Read the model definition and answer for the solid it produces. Units are mm, in the model's axes. A direction names the side the tool comes from. Give positions to 0.01 mm unless a question says otherwise; leave off trailing zeros. Loops run counter-clockwise (first coordinate to the right, second up) from the corner with the lowest first, then second, coordinate; pieces in that order, holes last. Notation, with made-up numbers: (30, -15) - (79, -15) arc R28 ccw to (79, 4) - close; hole circle Ø1 at (75, -10.5). An arc over 180 degrees is marked (long way). Use a Markdown table: item, result. Add a question column.
Item 1: A cutting plane is placed at B-B (x = 0). Determine the outline of the cut face in (y, z).
Item 2: Which of the six approach directions +Z, -Z, +X, -X, +Y, -Y give full straight-line access (tool end or side, diameter ignored) to faces 4 (the face through (0, -5, 17)), 5 (the face through (-2.3, -2.2, -15.7)), 6 (the face through (0, -1, -25)), 7 (the face through (8.5, -9.7, -12)), 8 (the face through (-10.43, -9.64, -11.4))?
Item 3: For a pull along Z with two mould halves and no side action, classify faces 1 (the face through (0, -10, -12)), 2 (the face through (9.797, -1.338, -23.859)), 3 (the face through (-11, -5, 5)) as +Z half, -Z half, draft (parallel to the pull), parting line (faces both ways), or undercut.
Item 4: A cutting plane is placed at D-D (y = -5.5). Determine the outline of the cut face in (x, z) (3 decimals).
Item 5: Each of these flat-tipped pins is pushed along its axis until it touches: P1, Ø2, axis at x = 1.5, y = -3.5, coming from the -Z side; P2, Ø0.5, axis at y = -10, z = -17, coming from the +X side; P3, Ø6, axis at x = 4, y = -5.5, coming from the +Z side; P4, Ø1.4, axis at y = -10, z = -18.5, coming from the -X side. Where does it stop, or does it pass through?
Item 6: A cutting plane is placed at A-A (z = 10.5). Determine the outline of the cut face in (x, y).
Item 7: Consider probe 1 along X at (y, z) = (-9.7, -18); probe 2 along X at (y, z) = (-8, 8.5); probe 3 along Y at (x, z) = (-4, 23.25). Determine where each line is inside the solid, lowest interval first. Write a range as [from, to].
Item 8: A cutting plane is placed at C-C (z = -18). Determine the outline of the cut face in (x, y).
from build123d import *

# Parameters (mm, degrees)
SALIENTE_EXTRUIR1_DEPTH         = 11
DI_METRO_DE_TALADRO_6_0_6_1_D   = 6
CORTAR_EXTRUIR1_DEPTH           = 36.071355834
CROQUIS6_W                      = 4.933877459
CROQUIS6_H                      = 16.455327893
CROQUIS6_W_2                    = 4.832675104
CORTAR_EXTRUIR5_DEPTH           = 4
REDONDEO1_R                     = 4
REDONDEO2_R                     = 4
REDONDEO3_R                     = 2
REDONDEO4_R                     = 0.5
DI_METRO_DE_TALADRO_6_4_6_4_1_D = 6.4


with BuildPart() as part:
    # Croquis1 → Saliente-Extruir1 (new body)
    with BuildSketch(Plane(origin=(0, 0, 0), x_dir=(1, 0, 0), z_dir=(0, 1, 0))):
        with BuildLine():
            Line((-7, 25), (7, 25))
            ThreePointArc((7, 25), (9.828427125, 23.828427125), (11, 21))
            Line((11, 21), (11, -21))
            ThreePointArc((11, -21), (9.828427125, -23.828427125), (7, -25))
            Line((7, -25), (-7, -25))
            ThreePointArc((-7, -25), (-9.828427125, -23.828427125), (-11, -21))
            Line((-11, -21), (-11, 21))
            ThreePointArc((-11, 21), (-9.828427125, 23.828427125), (-7, 25))
        make_face()
        with BuildLine():
            Line((-8, -17), (8, -17))
            Line((8, -17), (8, 4))
            ThreePointArc((8, 4), (0, 12), (-8, 4))
            Line((-8, 4), (-8, -17))
        make_face(mode=Mode.SUBTRACT)
    extrude(amount=-SALIENTE_EXTRUIR1_DEPTH)

    # Diámetro de taladro Ø6.0 (6)1 (through all)
    with Locations(Plane(origin=(0, 0, 0), x_dir=(1, 0, 0), z_dir=(0, 1, 0))):
        with Locations((0, 18)):
            Hole(DI_METRO_DE_TALADRO_6_0_6_1_D / 2)

    # Croquis5 → Cortar-Extruir1 (cut, through all)
    with BuildSketch(Plane(origin=(11, 0, 0), x_dir=(0, 0, -1), z_dir=(1, 0, 0))):
        with BuildLine():
            Line((6.7, -2.2), (26.063321608, -2.2))
            Line((26.063321608, -2.2), (26.063321608, -8.8))
            Line((26.063321608, -8.8), (6.7, -8.8))
            ThreePointArc((6.7, -8.8), (3.4, -5.5), (6.7, -2.2))
        make_face()
    extrude(amount=-CORTAR_EXTRUIR1_DEPTH, mode=Mode.SUBTRACT)

    # Croquis6 → Cortar-Extruir5 (cut)
    with BuildSketch(Plane.XZ.offset(11)):
        with Locations((10.46693873, -20.227663947)):
            Rectangle(CROQUIS6_W, CROQUIS6_H)
        with Locations((-10.416337552, -20.227663947)):
            Rectangle(CROQUIS6_W_2, CROQUIS6_H)
    extrude(amount=-CORTAR_EXTRUIR5_DEPTH, mode=Mode.SUBTRACT)

    # Redondeo1
    # the kernel refuses this fillet: 4 mm, written as the material it takes off along each edge
    with BuildSketch(Plane(origin=(8, -21.005040364, -24.872983346), x_dir=(-0.9994962175029386, 0, -0.031738166256391975), z_dir=(0, 1, 0))) as redondeo1_piece_1:
        with BuildLine():
            CenterArc((3.875063481, 3.99798487), REDONDEO1_R, 181.818768407, 90)
            Line((-0.122921389, 3.871032205), (-0.522719876, 3.858336938))
            Line((-0.522719876, 3.858336938), (-0.399798487, -0.012695267))
            Line((-0.399798487, -0.012695267), (-0.087657483, -0.390277037))
            ThreePointArc((-0.087657483, -0.390277037), (1.01622276, -0.495012986), (4.014711412, -0.399798487))
            Line((4.014711412, -0.399798487), (4.002016146, 0))
        make_face()
    extrude(amount=12.205040364, mode=Mode.SUBTRACT)

    # Redondeo2
    # the kernel refuses this fillet: 4 mm, written as the material it takes off along each edge
    with BuildSketch(Plane(origin=(-8, -21.005040364, -24.872983346), x_dir=(0, 0, 1), z_dir=(0, 1, 0))) as redondeo2_piece_1:
        with BuildLine():
            CenterArc((3.872983346, 4), REDONDEO2_R, 180, 90)
            Line((-0.127016654, 4), (-0.527016654, 4))
            ThreePointArc((-0.527016654, 4), (-0.527016654, 1), (-0.387298335, -0.1))
            Line((-0.387298335, -0.1), (0, -0.4))
            Line((0, -0.4), (3.872983346, -0.4))
            Line((3.872983346, -0.4), (3.872983346, 0))
        make_face()
    extrude(amount=12.205040364, mode=Mode.SUBTRACT)

    # Redondeo3
    redondeo3_edges = [part.edges().sort_by_distance(p)[0] for p in [
        (-11, -9.9, -12),
        (11, -9.9, -12),
    ]]
    fillet(redondeo3_edges, radius=REDONDEO3_R)

    # Redondeo4
    redondeo4_edges = [part.edges().sort_by_distance(p)[0] for p in [
        (9.828427125, -11, 23.828427125),
        (0, 0, 25),
        (-9.828427125, 0, 23.828427125),
        (-8.5, -11, -12),
        (0, -11, -25),
        (6.828427125, -11, -23.828427125),
        (-8, -11, -16.5),
        (11, -11, 5.5),
        (-6.828427125, -11, -23.828427125),
        (-11, -11, 5.5),
        (8.5, -11, -12),
        (10.414213562, -11, -11.414213562),
        (-10.414213562, -11, -11.414213562),
        (-9.828427125, -11, 23.828427125),
        (0, -11, 25),
        (-11, 0, 0),
        (-9.828427125, 0, -23.828427125),
        (0, 0, -25),
        (8, -11, -16.5),
        (9.828427125, 0, -23.828427125),
        (11, 0, 0),
        (9.828427125, 0, 23.828427125),
    ]]
    fillet(redondeo4_edges, radius=REDONDEO4_R)

    # Diámetro de taladro Ø6.4 (6.4)1 (through all)
    with Locations(Plane.XY.offset(25)):
        with Locations((-4, -5.5), (4, -5.5)):
            Hole(DI_METRO_DE_TALADRO_6_4_6_4_1_D / 2)


solid = part.part
Geometry says:
| question | item | result |
|---|---|---|
| 1 | outline | (-11, -24.5) arc R0.5 ccw to (-10.5, -25) - (-8.8, -25) - (-8.8, -21) - (-11, -21) - close; (-11, -15) - (-8.8, -15) - (-8.8, -12) - (-11, -12) - close; (-11, 17) - (0, 17) - (0, 24.5) arc R0.5 ccw to (-0.5, 25) - (-10.5, 25) arc R0.5 ccw to (-11, 24.5) - close; (-2.2, -25) - (-0.5, -25) arc R0.5 ccw to (0, -24.5) - (0, -21) - (-2.2, -21) - close; (-2.2, -15) - (0, -15) - (0, -12) - (-2.2, -12) - close |
| 2 | face 4 | +Y, -Y |
| 2 | face 5 | -Z, +X, -X |
| 2 | face 6 | -Z, +X, -X, +Y, -Y |
| 2 | face 7 | -Z, +X, -Y |
| 2 | face 8 | -Z, -X, -Y |
| 3 | face 1 | undercut |
| 3 | face 2 | -Z half |
| 3 | face 3 | draft |
| 4 | outline | (-11, -3.4) - (-8, -3.4) - (-8, 17) - (-7.2, 17) - (-7.2, 24.995) arc R4 ccw to (-11, 21) - close; (-0.8, 17) - (0.8, 17) - (0.8, 25) - (-0.8, 25) - close; (7.2, 17) - (8, 17) - (8, -3.4) - (11, -3.4) - (11, 21) arc R4 ccw to (7.2, 24.995) - close |
| 5 | P1 | z = 17 |
| 5 | P2 | x = 8 |
| 5 | P3 | through |
| 5 | P4 | x = -8 |
| 6 | outline | (-11, -10.5) arc R0.5 ccw to (-10.5, -11) - (-8, -11) - (-8, 0) - (-10.5, 0) arc R0.5 ccw to (-11, -0.5) - close; (8, -11) - (10.5, -11) arc R0.5 ccw to (11, -10.5) - (11, -0.5) arc R0.5 ccw to (10.5, 0) - (8, 0) - close |
| 7 | probe 1 | [-8, -3], [3, 8] |
| 7 | probe 2 | [-11, -8], [8, 11] |
| 7 | probe 3 | [-11, -8.7], [-2.3, 0] |
| 8 | outline | (-11, -2.2) - (-3, -2.2) - (-3, 0) - (-10.5, 0) arc R0.5 ccw to (-11, -0.5) - close; (-8, -10.5) arc R0.5 ccw to (-7.5, -11) - (-3, -11) - (-3, -8.8) - (-8, -8.8) - close; (3, -11) - (7.5, -11) arc R0.5 ccw to (8, -10.5) - (8, -8.8) - (3, -8.8) - close; (3, -2.2) - (11, -2.2) - (11, -0.5) arc R0.5 ccw to (10.5, 0) - (3, 0) - close |
